Geometry check sheet. Reference: drawing and pictorial views, mm from the part's lowest x, y, z. A direction names the side the tool comes from. Round coordinates to 2 decimals unless told otherwise and drop trailing zeros. Loops run counter-clockwise (first coordinate to the right, second up) from the corner with the lowest first, then second, coordinate; pieces in that order, holes last. Notation, with made-up numbers: (15, -8.75) -> (20, -8.75) arc R29 cw to (20, 22.25) -> close; hole circle Ø4 at (32, -13). An arc over 180 degrees is marked (long way). Use one line per item in the form item = value. Start each with the question number.
(1) Sectioned sample at B-B (y = 33.5). Record the cut outline in (x, z).
(2) Go/stop test with flat-tipped pins: pin 1 (12 mm diameter, centred on x = 64, z = 24, fed in from -Y); pin 2 (20.5 mm diameter, centred on y = 28.575, z = 57.15, fed in from +X). Record where each tip stops, or that it passes through.
(3) Sectioned sample at C-C (z = 57.15). Record the cut outline in (x, y) (1 decimal).
(4) Set-up check for the marked faces 5 and 6: record each of +Z, -Z, +X, -X, +Y, -Y from which the full face is reachable in a straight line by a thin tool's end or side.
(5) Draft check along Y on the marked faces 1, 2, 3 and 4. Enter one of: released by +Y, released by -Y, zero draft, split by the parting line, or undercut.
(6) Sectioned sample at D-D (x = 122.5). Record the cut outline in (y, z).
(7) Material ranges on probe 1 along Y at (x, z) = (127, 4.75); probe 2 along Z at (x, y) = (29, 13); probe 3 along X at (y, z) = (51.5, 26), recorded low to high. Write a range as [from, to].
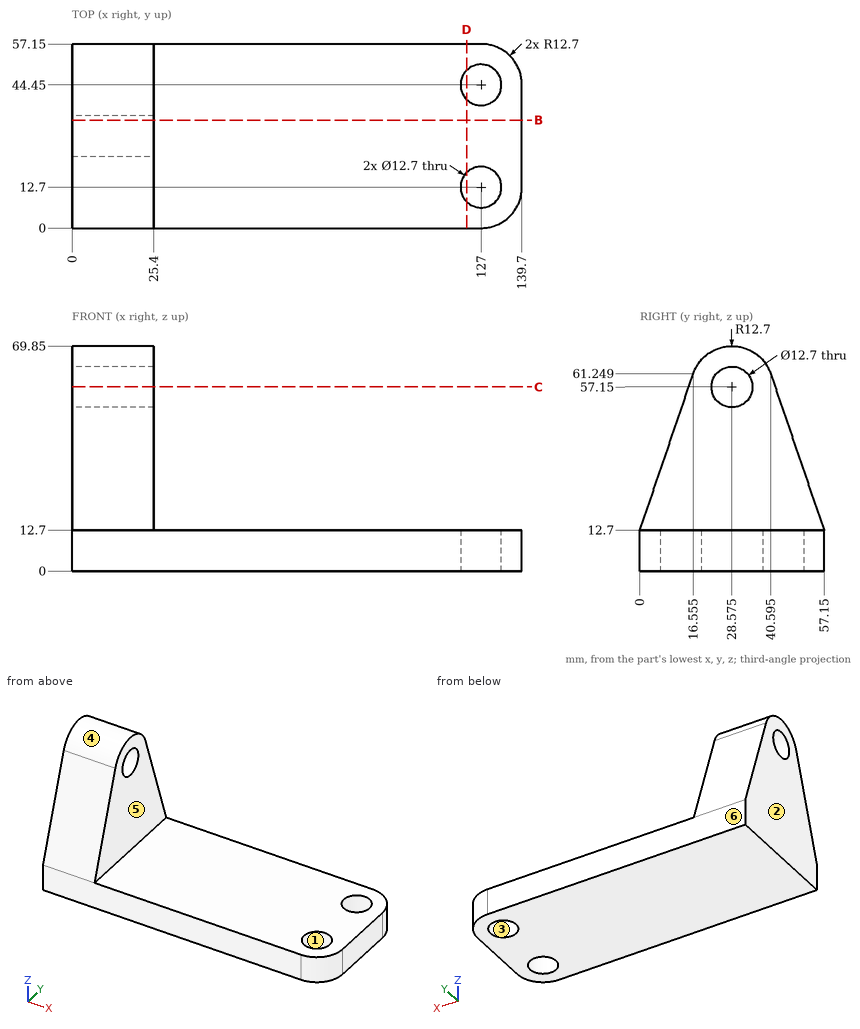
Checks:
q1.outline = (0, 0) -> (139.7, 0) -> (139.7, 12.7) -> (25.4, 12.7) -> (25.4, 53.14) -> (0, 53.14) -> close; (0, 61.16) -> (25.4, 61.16) -> (25.4, 68.86) -> (0, 68.86) -> close
q2.pin_1 = through
q2.pin_2 = 25.4
q3.outline = (0, 15.2) -> (25.4, 15.2) -> (25.4, 22.2) -> (0, 22.2) -> close; (0, 34.9) -> (25.4, 34.9) -> (25.4, 42) -> (0, 42) -> close
q4.face_5 = +Z, +X, +Y, -Y
q4.face_6 = +Z, -Z, +X, -X, +Y
q5.face_1 = undercut
q5.face_2 = zero draft
q5.face_3 = undercut
q5.face_4 = split by the parting line
q6.outline = (0, 0) -> (8.22, 0) -> (8.22, 12.7) -> (0, 12.7) -> close; (17.18, 0) -> (39.97, 0) -> (39.97, 12.7) -> (17.18, 12.7) -> close; (48.93, 0) -> (57.15, 0) -> (57.15, 12.7) -> (48.93, 12.7) -> close
q7.probe_1 = [0, 6.35], [19.05, 38.1], [50.8, 57.15]
q7.probe_2 = [0, 12.7]
q7.probe_3 = [0, 25.4]
